```python
from build123d import *

# Parameters (mm, degrees)
SKETCH1_W            = 63.5
SKETCH1_H            = 44.45
SKETCH1_W_2          = 32.512
SKETCH1_H_2          = 13.716
BOSS_EXTRUDE1_DEPTH  = 40.005
SKETCH2_W            = 32.512
SKETCH2_H            = 13.716
BOSS_EXTRUDE2_DEPTH  = 2.54
CUT_EXTRUDE1_DEPTH   = 36.83
BOSS_EXTRUDE8_DEPTH  = 6.35
BOSS_EXTRUDE9_REACH  = 92.627
SKETCH10_W           = 21.463
SKETCH10_H           = 3.175
SKETCH11_W           = 9.0805
SKETCH11_H           = 36.83
CUT_EXTRUDE2_DEPTH   = 88.226443955
SKETCH12_W           = 21.463
SKETCH12_H           = 30.48
SKETCH12_R           = 5.08
BOSS_EXTRUDE10_DEPTH = 2.54
SKETCH13_W           = 24.638
SKETCH13_H           = 35.3695
BOSS_EXTRUDE11_DEPTH = 3.175
SKETCH14_R           = 5.08
CUT_EXTRUDE3_DEPTH   = 6.35


with BuildPart() as part:
    # Sketch1 → Boss-Extrude1 (new body)
    with BuildSketch(Plane(origin=(0, 0, 0), x_dir=(1, 0, 0), z_dir=(0, 1, 0))):
        with Locations((31.75, 22.225)):
            Rectangle(SKETCH1_W, SKETCH1_H)
        with Locations((19.431, 25.3365)):
            Rectangle(SKETCH1_W_2, SKETCH1_H_2, mode=Mode.SUBTRACT)
        with Locations((19.431, 10.033)):
            Rectangle(SKETCH1_W_2, SKETCH1_H_2, mode=Mode.SUBTRACT)
    extrude(amount=BOSS_EXTRUDE1_DEPTH)

    # Sketch2 → Boss-Extrude2 (add)
    with BuildSketch(Plane.XZ):
        with Locations((19.431, -10.033)):
            Rectangle(SKETCH2_W, SKETCH2_H)
        with Locations((19.431, -25.3365)):
            Rectangle(SKETCH2_W, SKETCH2_H)
    extrude(amount=-BOSS_EXTRUDE2_DEPTH)

    # Sketch3 → Cut-Extrude1 (cut)
    with BuildSketch(Plane(origin=(0, 40.005, 0), x_dir=(1, 0, 0), z_dir=(0, 1, 0))):
        Polygon((3.175, 35.3695), (35.687, 35.3695), (38.862, 35.3695), (38.862, 32.1945), (38.862, 18.4785), (38.862, 0), (63.5, 0), (63.5, 44.45), (0, 44.45), (0, 35.3695), align=None)
    extrude(amount=-CUT_EXTRUDE1_DEPTH, mode=Mode.SUBTRACT)

    # Sketch9 → Boss-Extrude8 (add)
    with BuildSketch(Plane.XY):
        Polygon((38.862, 36.83), (0, 36.83), (0, 0), (63.5, 0), (63.5, 3.175), (38.862, 3.175), align=None)
    extrude(amount=BOSS_EXTRUDE8_DEPTH)

    # Boss-Extrude9: up to this face of the body (flat: up to its plane)
    boss_extrude9_end = Plane(part.part.faces().sort_by_distance((31.75, 1.5875, -44.45))[0])
    # Sketch10 → Boss-Extrude9 (add, up to the picked face)
    with BuildSketch(Plane.XY.offset(6.35), mode=Mode.PRIVATE) as boss_extrude9_sk1:
        Polygon((60.325, 3.175), (63.5, 3.175), (63.5, 36.83), (60.325, 36.83), (60.325, 33.655), (60.325, 30.48), align=None)
    boss_extrude9_tool1 = split(extrude(boss_extrude9_sk1.sketch, amount=-BOSS_EXTRUDE9_REACH, mode=Mode.PRIVATE), bisect_by=boss_extrude9_end, keep=Keep.BOTH, mode=Mode.PRIVATE)
    # Sketch10 → Boss-Extrude9 (add, up to the picked face)
    with BuildSketch(Plane.XY.offset(6.35), mode=Mode.PRIVATE) as boss_extrude9_sk2:
        with Locations((49.5935, 35.2425)):
            Rectangle(SKETCH10_W, SKETCH10_H)
    boss_extrude9_tool2 = split(extrude(boss_extrude9_sk2.sketch, amount=-BOSS_EXTRUDE9_REACH, mode=Mode.PRIVATE), bisect_by=boss_extrude9_end, keep=Keep.BOTH, mode=Mode.PRIVATE)
    add(boss_extrude9_tool1.solids().sort_by(Axis((61.9125, 20.0025, 6.35), (0, 0, -1)))[0])
    add(boss_extrude9_tool2.solids().sort_by(Axis((49.5935, 35.2425, 6.35), (0, 0, -1)))[0])

    # Sketch11 → Cut-Extrude2 (cut, through all)
    with BuildSketch(Plane.ZY):
        with Locations((-39.90975, 18.415)):
            Rectangle(SKETCH11_W, SKETCH11_H)
    extrude(amount=-CUT_EXTRUDE2_DEPTH, mode=Mode.SUBTRACT)

    # Sketch12 → Boss-Extrude10 (add)
    with BuildSketch(Plane(origin=(0, 0, -35.3695), x_dir=(-1, 0, 0), z_dir=(0, 0, -1))):
        with Locations((-49.5935, 18.415)):
            Rectangle(SKETCH12_W, SKETCH12_H)
        with Locations((-49.5935, 18.415)):
            Circle(SKETCH12_R, mode=Mode.SUBTRACT)
    extrude(amount=-BOSS_EXTRUDE10_DEPTH)

    # Sketch13 → Boss-Extrude11 (add)
    with BuildSketch(Plane(origin=(0, 36.83, 0), x_dir=(1, 0, 0), z_dir=(0, 1, 0))):
        with Locations((51.181, 17.68475)):
            Rectangle(SKETCH13_W, SKETCH13_H)
    extrude(amount=BOSS_EXTRUDE11_DEPTH)

    # Sketch14 → Cut-Extrude3 (cut)
    with BuildSketch(Plane(origin=(0, 40.005, 0), x_dir=(1, 0, 0), z_dir=(0, 1, 0))):
        with Locations(Location((49.5935, 17.68475, 0), (0, 0, 270))):
            Circle(SKETCH14_R)
    extrude(amount=-CUT_EXTRUDE3_DEPTH, mode=Mode.SUBTRACT)


solid = part.part
```
Source: CAD feature listing. Evaluate the final solid. Frame: model axes, mm. A direction names the side the tool comes from. Coordinates: 2 decimals unless noted, no trailing zeros. Write each loop counter-clockwise with the first axis right and the second up, starting at its lowest first coordinate (ties: lowest second). Pieces come first, ordered by that corner, then holes. Notation, with made-up numbers: (40, 49.5) -> (76, 49.5) arc R4 ccw to (76, 53.5) -> close; hole circle Ø8 at (29.25, 70.25). An arc over 180 degrees is marked (long way). Return JSON: item names as keys, results as strings. Group by question number.
1) Mould query, pull axis X, two halves, no side actions, for faces 1 (the face through (31, 0, -15)), 2 (the face through (19, 21, -3.175)), 3 (the face through (63.5, 20, -14)). Classes: +X half, -X half, draft (parallel to the pull), parting line (faces both ways), or undercut.
2) Ray query, line 1 along X through (y, z) = (32, -26.5) (3 decimals); line 2 along X through (y, z) = (36, -18); line 3 along X through (y, z) = (20, 0.5) (3 decimals). Return the intervals inside material, ascending.
3) Section query B-B, the plane z = -1. Return loops of the section in (x, y) (3 decimals), plus the area to 3 significant figures.
4) Set-up query: faces 4 (the face through (31, 40.005, -18)), 5 (the face through (38.862, 18, -14)), 6 (the face through (31, 38, 0)), 7 (the face through (35.687, 21, -10)). Return all of +Z, -Z, +X, -X, +Y, -Y with unobstructed straight access to the full face (end or side cutting, diameter ignored); none if empty.
5) Section query A-A, the plane y = 19.5. State how many separate pieces and enclosed holes the cut face has, plus the area to 3 significant figures.
6) Contact query for flat-ended pins moving along their axis: P1, Ø8, axis at x = 49.59, y = 18.42, coming from the +Z side; P2, Ø1.9, axis at x = 19.5, z = 4.5, coming from the +Y side; P3, Ø2.5, axis at x = 22, y = 38.5, coming from the +Z side; P4, Ø2, axis at x = 13, z = -29, coming from the +Y side. Output: stop coordinate, or through.
From the geometry:
{
 "1": {"face 1": "draft", "face 2": "undercut", "face 3": "+X half"},
 "2": {"line 1": "0 to 3.175, 35.687 to 38.862, 60.325 to 63.5", "line 2": "0 to 44.52, 54.66 to 63.5", "line 3": "0 to 38.862, 60.325 to 63.5"},
 "3": {"outline": "(0, 0) -> (63.5, 0) -> (63.5, 40.005) -> (0, 40.005) -> close; hole (38.862, 3.175) -> (60.325, 3.175) -> (60.325, 33.655) -> (38.862, 33.655) -> close", "area": "1,890 mm²"},
 "4": {"face 4": "+Z, -Z, +X, -X, +Y", "face 5": "+Z", "face 6": "+Z, +X, -X, +Y", "face 7": "+Y"},
 "5": {"separate pieces": "2", "enclosed holes": "2", "area": "891 mm²"},
 "6": {"P1": "through", "P2": "y = 36.83", "P3": "z = 0", "P4": "y = 2.54"}
}
